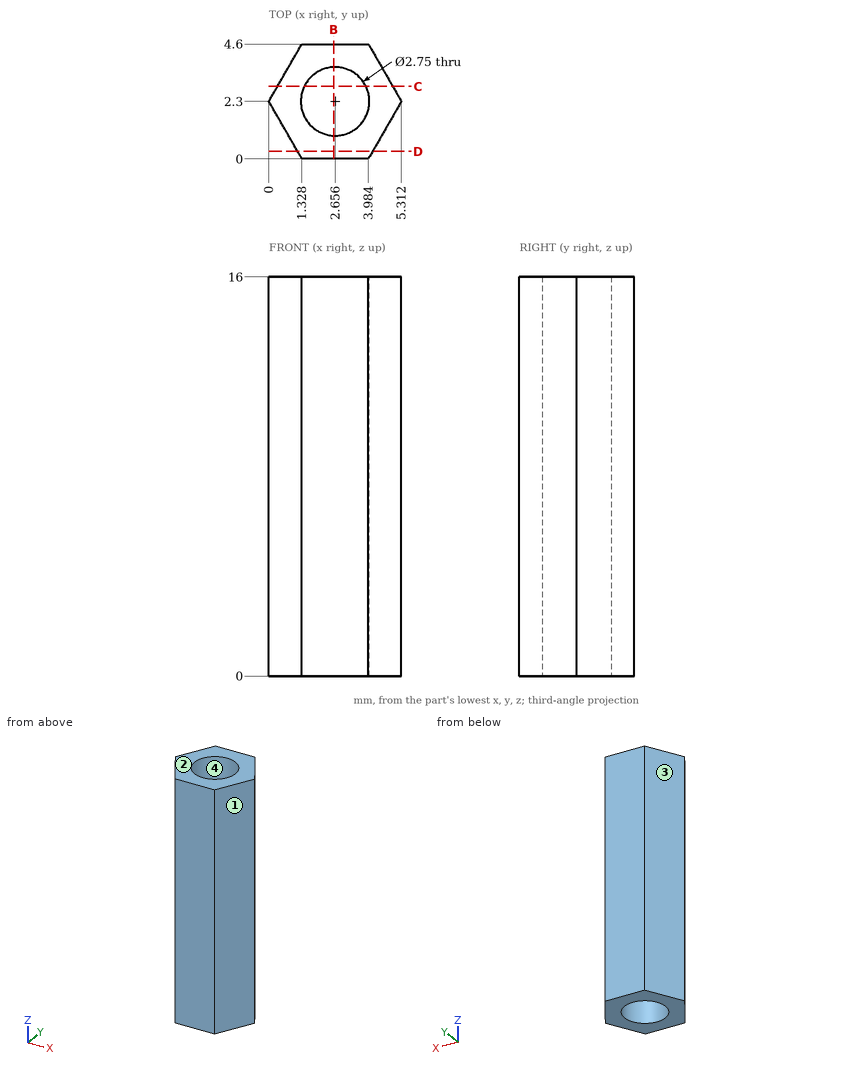
Geometry check sheet. Reference: drawing and pictorial views, mm from the part's lowest x, y, z. Round coordinates to 2 decimals unless told otherwise and drop trailing zeros. Loops run counter-clockwise (first coordinate to the right, second up) from the corner with the lowest first, then second, coordinate; pieces in that order, holes last. Notation, with made-up numbers: (64.5, -37.75) - (119.5, -37.75) arc R27 ccw to (119.5, -17.75) - close; hole circle Ø6 at (-21.75, 17.25). An arc over 180 degrees is marked (long way). Use a Markdown table: item, result. Add a question column.
1. Thickness scan on probe 1 along Y at (x, z) = (2.6, 4.25); probe 2 along Y at (x, z) = (1.8, 1.25) (1 decimal); probe 3 along X at (y, z) = (2.25, 15.25). Record the ranges inside material, lowest first. Write a range as [from, to].
2. Gauge pin test, flat end, axial feed: pin 1 (1 mm diameter, centred on y = 3.5, z = 2.5, fed in from -X). Record the tip position at first contact, or that the pin passes through.
3. Release check for a two-part mould opening along Y. For the marked faces 1, 2, 3 and 4 record: released by +Y, released by -Y, zero draft, split by the parting line, or undercut.
4. Section check C-C, the plane y = 2.9. Record the boundary of the cut face in (x, z) (1 decimal).
5. Section check B-B, the plane x = 2.6. Record the boundary of the cut face in (y, z).
6. Section check D-D, the plane y = 0.3. Record the boundary of the cut face in (x, z) (1 decimal).
Checks:
| question | item | result |
|---|---|---|
| 1 | probe 1 | y = [0, 0.93], [3.67, 4.6] |
| 1 | probe 2 | y = [0, 1.2], [3.4, 4.6] |
| 1 | probe 3 | x = [0.03, 1.28], [4.03, 5.28] |
| 2 | pin 1 | stops at x = 0.4 |
| 3 | face 1 | released by -Y |
| 3 | face 2 | zero draft |
| 3 | face 3 | released by +Y |
| 3 | face 4 | undercut |
| 4 | outline | (0.3, 0) - (1.4, 0) - (1.4, 16) - (0.3, 16) - close; (3.9, 0) - (5, 0) - (5, 16) - (3.9, 16) - close |
| 5 | outline | (0, 0) - (0.93, 0) - (0.93, 16) - (0, 16) - close; (3.67, 0) - (4.6, 0) - (4.6, 16) - (3.67, 16) - close |
| 6 | outline | (1.2, 0) - (4.2, 0) - (4.2, 16) - (1.2, 16) - close |
